Design review of the part built by this model. Coordinates are the model's own, in mm. A direction names the side the tool comes from. Give positions to 0.01 mm unless a question says otherwise; leave off trailing zeros. Write each loop counter-clockwise with the first axis right and the second up, starting at its lowest first coordinate (ties: lowest second). Pieces come first, ordered by that corner, then holes. Notation, with made-up numbers: M -30.5,75.5 L 16.5,75.5 A16 cw 16.5,103.5 Z; hole C 7,-11 d9. An arc over 180 degrees is marked long. Answer in a Markdown table with one row per item.
```python
from build123d import *

# Parameters (mm, degrees)
BASE_EXTRUDE_DEPTH      = 6
SKETCH5_W               = 6.5
SKETCH5_H               = 12
CUT_EXTRUDE3_DEPTH      = 6
CUT_EXTRUDE3_DEPTH_BACK = 10
SKETCH7_R               = 2.5
CUT_EXTRUDE4_DEPTH      = 11
CHAMFER2_SIZE           = 0.2
SKETCH6_R               = 2.5
CUT_EXTRUDE5_DEPTH      = 7
CUT_EXTRUDE5_DEPTH_BACK = 7


with BuildPart() as part:
    # Sketch2 → Base-Extrude (new body, symmetric)
    with BuildSketch(Plane.XY):
        with BuildLine():
            Line((-18, 6), (3.392304845, 6))
            ThreePointArc((3.392304845, 6), (5, 0), (3.392304845, -6))
            Line((3.392304845, -6), (-18, -6))
            Line((-18, -6), (-18, 6))
        make_face()
    extrude(amount=BASE_EXTRUDE_DEPTH, both=True)

    # Sketch5 → Cut-Extrude3 (cut, two sides)
    with BuildSketch(Plane(origin=(0, 0, 0), x_dir=(0, 0, -1), z_dir=(1, 0, 0))) as cut_extrude3_sk:
        Rectangle(SKETCH5_W, SKETCH5_H)
    extrude(amount=CUT_EXTRUDE3_DEPTH, mode=Mode.SUBTRACT)
    extrude(cut_extrude3_sk.sketch, amount=-CUT_EXTRUDE3_DEPTH_BACK, mode=Mode.SUBTRACT)

    # Sketch7 → Cut-Extrude4 (cut)
    with BuildSketch(Plane.ZY.offset(18)):
        Circle(SKETCH7_R)
    extrude(amount=-CUT_EXTRUDE4_DEPTH, mode=Mode.SUBTRACT)

    # Chamfer2
    chamfer2_edges = [part.edges().sort_by_distance(p)[0] for p in [
        (-18, 0, -2.5),
    ]]
    chamfer(chamfer2_edges, length=CHAMFER2_SIZE)

    # Sketch6 → Cut-Extrude5 (cut, two sides)
    with BuildSketch(Plane.XY) as cut_extrude5_sk:
        Circle(SKETCH6_R)
    extrude(amount=CUT_EXTRUDE5_DEPTH, mode=Mode.SUBTRACT)
    extrude(cut_extrude5_sk.sketch, amount=-CUT_EXTRUDE5_DEPTH_BACK, mode=Mode.SUBTRACT)


solid = part.part
```
1) Add section A-A (x = -5). Write out the cut boundary in (y, z).
Geometry says:
| item | result |
|---|---|
| outline | M -6,-6 L 6,-6 L 6,-3.25 L -6,-3.25 Z; M -6,3.25 L 6,3.25 L 6,6 L -6,6 Z |
2) The part is to be moulded in two halves that separate along Y. For faces 3 (the face through (-4, 0, -3.25)), 4 (the face through (-13.95, -2.44, -0.54)), 5 (the face through (5, 0, -5)), 6 (the face through (-12, 6, 0)), say which applies: released by +Y, released by -Y, zero draft, split by the parting line, or undercut.
Geometry says:
| item | result |
|---|---|
| face 3 | zero draft |
| face 4 | undercut |
| face 5 | split by the parting line |
| face 6 | released by +Y |
3) Add section C-C (x = 0). Write out the cut boundary in (y, z).
Geometry says:
| item | result |
|---|---|
| outline | M -6,-6 L -2.5,-6 L -2.5,-3.25 L -6,-3.25 Z; M -6,3.25 L -2.5,3.25 L -2.5,6 L -6,6 Z; M 2.5,-6 L 6,-6 L 6,-3.25 L 2.5,-3.25 Z; M 2.5,3.25 L 6,3.25 L 6,6 L 2.5,6 Z |
4) Insertion check: P1, Ø2, axis at y = -3, z = 0, coming from the +X side. The pin has a flat end and moves straight along its axis. Give the tip position at first contact, or say it passes through.
Geometry says:
| item | result |
|---|---|
| P1 | x = -10 |
5) Add section B-B (z = 0). Write out the cut boundary in (x, y).
Geometry says:
| item | result |
|---|---|
| outline | M -18,-6 L -10,-6 L -10,-2.5 L -17.8,-2.5 L -18,-2.7 Z; M -18,2.7 L -17.8,2.5 L -10,2.5 L -10,6 L -18,6 Z |
6) For faces 1 (the face through (-10, 3, 0)), 2 (the face through (-0.54, -2.44, -4.61)), list the 3-axis set-ups (+Z, -Z, +X, -X, +Y, -Y) from which the entire face can be reached by the end or side of a thin tool; tool diameter is ignored.
Geometry says:
| item | result |
|---|---|
| face 1 | +X, +Y, -Y |
| face 2 | +Z, -Z |
7) Add section D-D (z = 5). Write out the cut boundary in (x, y), and give its area (3 significant figures).
Geometry says:
| item | result |
|---|---|
| outline | M -18,-6 L 3.39,-6 A12 ccw 3.39,6 L -18,6 Z; hole C 0,0 d5 |
| area | 250 mm^2 |
8) To check wall thickness, follow probe 1 along Y at (x, z) = (0, 5.25); probe 2 along Z at (x, y) = (-6.25, -0.5); probe 3 along X at (y, z) = (0, 4.8). State the ranges of each line that lie inside material, in increasing order. Write a range as [from, to].
Geometry says:
| item | result |
|---|---|
| probe 1 | [-6, -2.5], [2.5, 6] |
| probe 2 | [-6, -3.25], [3.25, 6] |
| probe 3 | [-18, -2.5], [2.5, 5] |
